Verification items for the finished model (mm, model axes). Round coordinates to 2 decimals unless told otherwise and drop trailing zeros. Order: outer loops, then holes, each group sorted by start corner. A loop starts at its lowest first (then second) coordinate and runs counter-clockwise, first axis right, second up. Notation, with made-up numbers: (4, 33.25) -> (46, 33.25) arc R10 cw to (46, 47.25) -> close; hole circle Ø5 at (-20.75, 51.5). An arc over 180 degrees is marked (long way). Return JSON: item names as keys, results as strings. Group by question number.
1) Section check A-A on x = 225. Enter the section's corners in (y, z).
2) Section check B-B on z = 1.65. State how many separate pieces and enclosed holes the cut face has, plus the area to 3 significant figures.
3) Depth check by flat-ended pin: pin 1 (1.8 mm diameter, centred on y = 94.5, z = 3, fed in from -X); pin 2 (1.8 mm diameter, centred on y = 93, z = 1.5, fed in from +X); pin 3 (3 mm diameter, centred on x = 51, z = 2.5, fed in from +Y). Enter the tip coordinate at first touch or a pass-through.
4) Section check C-C on y = -15. Enter the section's corners in (x, z).
5) Scan lines: L1, parallel to Y at x = -140, z = 4.95; L2, parallel to X at y = -4, z = 2.55. Record each from-to range of solid material in increasing order.
```python
from build123d import *

# Parameters (mm, degrees)
SKETCH1_W           = 790
SKETCH1_H           = 180
BOSS_EXTRUDE1_DEPTH = 6
SKETCH2_W           = 50
SKETCH2_H           = 6
SKETCH2_W_2         = 30
CUT_EXTRUDE1_DEPTH  = 10
SKETCH3_W           = 6
SKETCH3_H           = 20
CUT_EXTRUDE2_DEPTH  = 10
SKETCH4_W           = 30
SKETCH4_H           = 6
BOSS_EXTRUDE2_DEPTH = 6
SKETCH5_W           = 6
SKETCH5_H           = 30
SKETCH5_H_2         = 29
SKETCH5_H_3         = 24
SKETCH5_H_4         = 21
CUT_EXTRUDE3_DEPTH  = 6


with BuildPart() as part:
    # Sketch1 → Boss-Extrude1 (new body)
    with BuildSketch(Plane.XY):
        Rectangle(SKETCH1_W, SKETCH1_H)
    extrude(amount=BOSS_EXTRUDE1_DEPTH)

    # Sketch2 → Cut-Extrude1 (cut)
    with BuildSketch(Plane.XY.offset(6)):
        with Locations((150, 7)):
            Rectangle(SKETCH2_W, SKETCH2_H)
        with Locations((0, 7)):
            Rectangle(SKETCH2_W_2, SKETCH2_H)
        with Locations((70, 7)):
            Rectangle(SKETCH2_W, SKETCH2_H)
        with Locations((230, 7)):
            Rectangle(SKETCH2_W, SKETCH2_H)
        with Locations((310, 7)):
            Rectangle(SKETCH2_W, SKETCH2_H)
        with Locations((390, 7)):
            Rectangle(SKETCH2_W, SKETCH2_H)
        with Locations((-390, 7)):
            Rectangle(SKETCH2_W, SKETCH2_H)
        with Locations((-310, 7)):
            Rectangle(SKETCH2_W, SKETCH2_H)
        with Locations((-230, 7)):
            Rectangle(SKETCH2_W, SKETCH2_H)
        with Locations((-150, 7)):
            Rectangle(SKETCH2_W, SKETCH2_H)
        with Locations((-70, 7)):
            Rectangle(SKETCH2_W, SKETCH2_H)
    extrude(amount=-CUT_EXTRUDE1_DEPTH, mode=Mode.SUBTRACT)

    # Sketch3 → Cut-Extrude2 (cut)
    with BuildSketch(Plane.XY.offset(6)):
        with Locations((-66, 50)):
            Rectangle(SKETCH3_W, SKETCH3_H)
        with Locations((-182, 50)):
            Rectangle(SKETCH3_W, SKETCH3_H)
        with Locations((50, 50)):
            Rectangle(SKETCH3_W, SKETCH3_H)
        with Locations((166, 50)):
            Rectangle(SKETCH3_W, SKETCH3_H)
        with Locations((282, 50)):
            Rectangle(SKETCH3_W, SKETCH3_H)
    extrude(amount=-CUT_EXTRUDE2_DEPTH, mode=Mode.SUBTRACT)

    # Sketch4 → Boss-Extrude2 (add)
    with BuildSketch(Plane.XY.offset(6)):
        with Locations((110, 93)):
            Rectangle(SKETCH4_W, SKETCH4_H)
        with Locations((30, 93)):
            Rectangle(SKETCH4_W, SKETCH4_H)
        with Locations((190, 93)):
            Rectangle(SKETCH4_W, SKETCH4_H)
        with Locations((270, 93)):
            Rectangle(SKETCH4_W, SKETCH4_H)
        with Locations((350, 93)):
            Rectangle(SKETCH4_W, SKETCH4_H)
        with Locations((-350, 93)):
            Rectangle(SKETCH4_W, SKETCH4_H)
        with Locations((-270, 93)):
            Rectangle(SKETCH4_W, SKETCH4_H)
        with Locations((-190, 93)):
            Rectangle(SKETCH4_W, SKETCH4_H)
        with Locations((-30, 93)):
            Rectangle(SKETCH4_W, SKETCH4_H)
        with Locations((-110, 93)):
            Rectangle(SKETCH4_W, SKETCH4_H)
    extrude(amount=-BOSS_EXTRUDE2_DEPTH)

    # Sketch5 → Cut-Extrude3 (cut)
    with BuildSketch(Plane.XY.offset(6)):
        with Locations((392, -75)):
            Rectangle(SKETCH5_W, SKETCH5_H)
        with Locations((392, -10.5)):
            Rectangle(SKETCH5_W, SKETCH5_H_2)
        with Locations((392, 78)):
            Rectangle(SKETCH5_W, SKETCH5_H_3)
        with Locations((392, 20.5)):
            Rectangle(SKETCH5_W, SKETCH5_H_4)
        with Locations((-392, 20.5)):
            Rectangle(SKETCH5_W, SKETCH5_H_4)
        with Locations((-392, 78)):
            Rectangle(SKETCH5_W, SKETCH5_H_3)
        with Locations((-392, -10.5)):
            Rectangle(SKETCH5_W, SKETCH5_H_2)
        with Locations((-392, -75)):
            Rectangle(SKETCH5_W, SKETCH5_H)
    extrude(amount=-CUT_EXTRUDE3_DEPTH, mode=Mode.SUBTRACT)


solid = part.part
```
Check result:
{
 "1": {"outline": "(-90, 0) -> (4, 0) -> (4, 6) -> (-90, 6) -> close; (10, 0) -> (90, 0) -> (90, 6) -> (10, 6) -> close"},
 "2": {"separate pieces": "1", "enclosed holes": "14", "area": "139,000 mm^2"},
 "3": {"pin 1": "x = -365", "pin 2": "x = 365", "pin 3": "y = 90"},
 "4": {"outline": "(-389, 0) -> (389, 0) -> (389, 6) -> (-389, 6) -> close"},
 "5": {"L1": "-90 to 4, 10 to 90", "L2": "-389 to 389"}
}
